from build123d import *

# Parameters (mm, degrees)
F0_W     = 94
F0_H     = 30
F1_DEPTH = 28
F2_W     = 94
F2_H     = 1.5
F3_DEPTH = 6
F4_R     = 14.5
F6_DEPTH = 3
F7_R     = 5.99999


# Not quite as in the source:
# - a fillet or chamfer is up to 0.001 mm smaller than in the source, because OpenCascade refuses the exact size


with BuildPart() as f1:
    # F0 (on Top) → F1 (new body)
    with BuildSketch(Plane.XY):
        with Locations((47, -15)):
            Rectangle(F0_W, F0_H)
    extrude(amount=F1_DEPTH)

    # F2 (on face) → F3 (join)
    with BuildSketch(Plane(origin=(0, 0, 0), x_dir=(1, 0, 0), z_dir=(0, 0, -1))):
        with Locations((47, 0.75)):
            Rectangle(F2_W, F2_H)
        with Locations((47, 29.25)):
            Rectangle(F2_W, F2_H)
    extrude(amount=F3_DEPTH)

    # F4
    f4_edges = [f1.edges().sort_by_distance(p)[0] for p in [
        (47, 0, 28),
        (47, -30, 28),
    ]]
    fillet(f4_edges, radius=F4_R)

    # F5 (on face) → F6 (join)
    with BuildSketch(Plane.YZ.offset(94)):
        with BuildLine():
            Line((-5.5, 31), (-24.5, 31))
            Line((-24.5, 31), (-24.5, 25))
            Line((-24.5, 25), (-24.3317608663, 25))
            ThreePointArc((-24.3317608663, 25), (-20.1636895265, 27.2295302177), (-15.5, 28))
            Line((-15.5, 28), (-14.5, 28))
            ThreePointArc((-14.5, 28), (-9.8363104735, 27.2295302177), (-5.6682391337, 25))
            Line((-5.6682391337, 25), (-5.5, 25))
            Line((-5.5, 25), (-5.5, 31))
        make_face()
    extrude(amount=-F6_DEPTH)

    # F7 (radius 6 in the source; OpenCascade refuses exactly that, so slightly less here)
    f7_edges = [f1.edges().sort_by_distance(p)[0] for p in [
        (92.5, -24.5, 31),
        (92.5, -5.5, 31),
    ]]
    fillet(f7_edges, radius=F7_R)


solid = f1.part
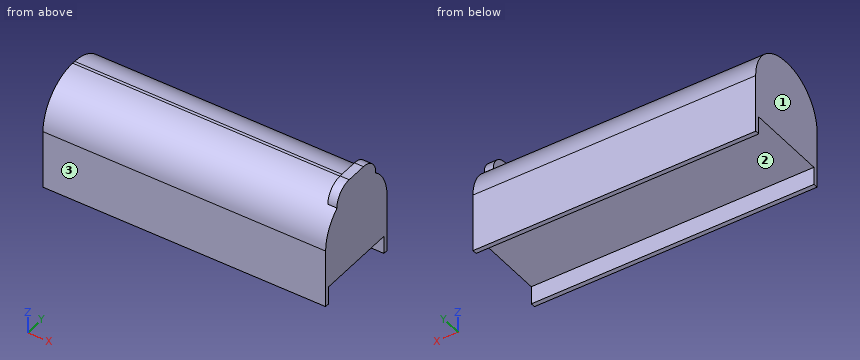
CAD build for the part. Positions are in the model's coordinates, mm. Face numbers are marked on the shaded views. Give positions to 0.01 mm unless a question says otherwise; leave off trailing zeros. Loops run counter-clockwise (first coordinate to the right, second up) from the corner with the lowest first, then second, coordinate; pieces in that order, holes last. Notation, with made-up numbers: M 47.5,62.25 L 81.5,62.25 A34 cw 81.5,98.25 Z; hole C 4.5,22.25 d6. An arc over 180 degrees is marked long. Answer in a Markdown table with one row per item. Add a question column.
Item 1: Band-saw the part on A-A on z = -1.5. Give the cut face in (x, y).
Item 2: Drop flat-ended pins along their axis: P1, Ø8, axis at x = 84, y = -13, coming from the +Z side; P2, Ø3, axis at x = 49, y = -21, coming from the -Z side; P3, Ø4, axis at x = 26, y = -22.5, coming from the +Z side. Give the stop position or say it passes through.
Item 3: Mould opens along Y. For the marked faces 1, 2 and 3 say: +Y half, -Y half, draft (parallel to the pull), parting line (faces both ways), or undercut.
Item 4: Band-saw the part on D-D on z = 21. Give the cut face in (x, y), then the cut area to 3 significant figures.
Item 5: Band-saw the part on C-C on y = -21.25. Give the cut face in (x, z), then the cut area to 3 significant figures.
Item 6: Probe probe 1 along Y at (x, z) = (21, -2.5); probe 2 along Y at (x, z) = (11, 25); probe 3 along Y at (x, z) = (70, 14.5). List the from-to ranges inside material, lowest first.
Item 7: Band-saw the part on B-B on x = 6.5. Give the cut face in (y, z), then the cut area to 3 significant figures.
Reply:
| question | item | result |
|---|---|---|
| 1 | outline | M 0,-30 L 94,-30 L 94,-28.5 L 0,-28.5 Z; M 0,-1.5 L 94,-1.5 L 94,0 L 0,0 Z |
| 2 | P1 | stops at z = 28 |
| 2 | P2 | stops at z = 0 |
| 2 | P3 | stops at z = 27.11 |
| 3 | face 1 | draft |
| 3 | face 2 | undercut |
| 3 | face 3 | -Y half |
| 4 | outline | M 0,-27.91 L 94,-27.91 L 94,-2.09 L 0,-2.09 Z |
| 4 | area | 2,430 mm^2 |
| 5 | outline | M 0,0 L 94,0 L 94,30.33 L 91,30.33 L 91,26.81 L 0,26.81 Z |
| 5 | area | 2,530 mm^2 |
| 6 | probe 1 | y = -30 to -28.5, -1.5 to 0 |
| 6 | probe 2 | y = -24.33 to -5.67 |
| 6 | probe 3 | y = -29.97 to -0.03 |
| 7 | outline | M -30,-6 L -28.5,-6 L -28.5,0 L -1.5,0 L -1.5,-6 L 0,-6 L 0,13.5 A14.5 ccw -14.5,28 L -15.5,28 A14.5 ccw -30,13.5 Z |
| 7 | area | 768 mm^2 |
